```python
from build123d import *

# Parameters (mm, degrees)
SKETCH3_R             = 25
BOSS_EXTRUDE1_DEPTH   = 15
SKETCH4_R             = 32
BOSS_EXTRUDE2_DEPTH   = 6
BOSS_EXTRUDE3_DEPTH   = 3
FILLET1_R             = 5
FILLET2_R             = 5
SKETCH8_R             = 3
CUT_EXTRUDE1_DEPTH    = 3
BODY_MOVE_COPY1_ANGLE = 120
BODY_MOVE_COPY4_ANGLE = 90


with BuildPart() as part:
    # Sketch3 → Boss-Extrude1 (new body)
    with BuildSketch(Plane(origin=(0, 0, 0), x_dir=(1, 0, 0), z_dir=(0, 1, 0))):
        Circle(SKETCH3_R)
    extrude(amount=-BOSS_EXTRUDE1_DEPTH)

    # Sketch4 → Boss-Extrude2 (add)
    with BuildSketch(Plane.XZ.offset(15)):
        Circle(SKETCH4_R)
    extrude(amount=BOSS_EXTRUDE2_DEPTH)

    # Sketch6 → Boss-Extrude3 (add)
    with BuildSketch(Plane.XZ.offset(21)):
        Polygon((35, 0), (35, -55), (-35, -55), (-35, 55), (35, 55), align=None)
    extrude(amount=BOSS_EXTRUDE3_DEPTH)

    # Fillet1
    fillet1_edges = [part.edges().sort_by_distance(p)[0] for p in [
        (35, -22.5, 55),
    ]]
    fillet(fillet1_edges, radius=FILLET1_R)

    # Fillet2
    fillet2_edges = [part.edges().sort_by_distance(p)[0] for p in [
        (-35, -22.5, 55),
        (-35, -22.5, -55),
        (35, -22.5, -55),
    ]]
    fillet(fillet2_edges, radius=FILLET2_R)

    # Sketch8 → Cut-Extrude1 (cut)
    with BuildSketch(Plane.XZ.offset(24)):
        with Locations((26.758523595, -46)):
            Circle(SKETCH8_R)
        with Locations((-28.158970904, -46)):
            Circle(SKETCH8_R)
        with Locations((26.758523595, 46)):
            Circle(SKETCH8_R)
        with Locations((-28.320886722, 45.663145403)):
            Circle(SKETCH8_R)
    extrude(amount=-CUT_EXTRUDE1_DEPTH, mode=Mode.SUBTRACT)


with BuildPart() as part_1:
    # Body-Move_Copy1: moved
    add(part.part.rotate(Axis((0, 0, 0), (-0.577350269, -0.577350269, 0.577350269)), BODY_MOVE_COPY1_ANGLE))


with BuildPart() as part_2:
    # Body-Move_Copy2: moved
    add(part_1.part.moved(Location((0, 0, -24))))


with BuildPart() as part_3:
    # Body-Move_Copy3: moved
    add(part_2.part.moved(Location((0, 0, 99))))


with BuildPart() as part_4:
    # Body-Move_Copy4: moved
    add(part_3.part.rotate(Axis((0, 0, 0), (0, 0, 1)), BODY_MOVE_COPY4_ANGLE))


solid = part_4.part
```
CAD build for the part. Positions are in the model's coordinates, mm. A direction names the side the tool comes from. Give positions to 0.01 mm unless a question says otherwise; leave off trailing zeros. Loops run counter-clockwise (first coordinate to the right, second up) from the corner with the lowest first, then second, coordinate; pieces in that order, holes last. Notation, with made-up numbers: M -40,52.5 L -30,52.5 A33 ccw -30,89.5 Z; hole C 71.5,74.25 d11. An arc over 180 degrees is marked long. Use one line per item in the form item = value.
Item 1: Slice it at A-A (x = 0). List the corners of the cut face in (y, z), plus the area to 3 significant figures.
Determined:
outline = M -55,96 L -32,96 L -32,90 L -25,90 L -25,75 L 25,75 L 25,90 L 32,90 L 32,96 L 55,96 L 55,99 L -55,99 Z
area = 1,460 mm2
Item 2: Slice it at C-C (z = 93.5). List the corners of the cut face in (x, y), plus the area to 3 significant figures.
Determined:
outline = C 0,0 d64
area = 3,220 mm2
Item 3: Slice it at D-D (y = 29.5). List the corners of the cut face in (x, z).
Determined:
outline = M -35,96 L -12.4,96 L -12.4,90 L 12.4,90 L 12.4,96 L 35,96 L 35,99 L -35,99 Z
Item 4: Two-plate mould, pull along X, no slides. Class faces 3 (the face through (-34, -53, 98)), 4 (the face through (25.46, -46.56, 97.52)), 5 (the face through (0, 0, 75)), 6 (the face through (33, -54, 98)): pulls with the +X half, pulls with the -X half, needs draft (parallel to the pull), parting line crosses it, or undercut.
Determined:
face_3 = pulls with the -X half
face_4 = undercut
face_5 = needs draft
face_6 = pulls with the +X half
Item 5: Drill centre lines: probe 1 along X at (y, z) = (46, 97.9); probe 2 along Z at (x, y) = (31, 28.5); probe 3 along Z at (x, y) = (25.5, 8.5). Where is each one in solid material? Low to high. Write a range as from..to.
Determined:
probe_1 = -35..-29.76, -23.76..25.16, 31.16..35
probe_2 = 96..99
probe_3 = 90..99
Item 6: Slice it at B-B (y = 0). List the corners of the cut face in (x, z), plus the area to 3 significant figures.
Determined:
outline = M -35,96 L -32,96 L -32,90 L -25,90 L -25,75 L 25,75 L 25,90 L 32,90 L 32,96 L 35,96 L 35,99 L -35,99 Z
area = 1,340 mm2
Item 7: Which spindle directions (+Z, -Z, +X, -X, +Y, -Y) get a long thin tool onto all of the face, cutting with end or side? Do faces 1 (the face through (31, 11, 96)), 2 (the face through (0, -1, 99)). Say none if no direction does.
Determined:
face_1 = -Z
face_2 = +Z, +X, -X, +Y, -Y
Item 8: Flat gauge pins, fed straight in: pin 1 (6 mm diameter, centred on x = -11.5, z = 95, fed in from +Y); pin 2 (8 mm diameter, centred on y = -21, z = 78, fed in from +X); pin 3 (9.5 mm diameter, centred on x = -26.76, y = 46, fed in from -Z); pin 4 (10 mm diameter, centred on y = -6, z = 90.5, fed in from -X). Where does each tip first touch, or does it go through?
Determined:
pin_1 = 55
pin_2 = 18.33
pin_3 = 96
pin_4 = -31.98
